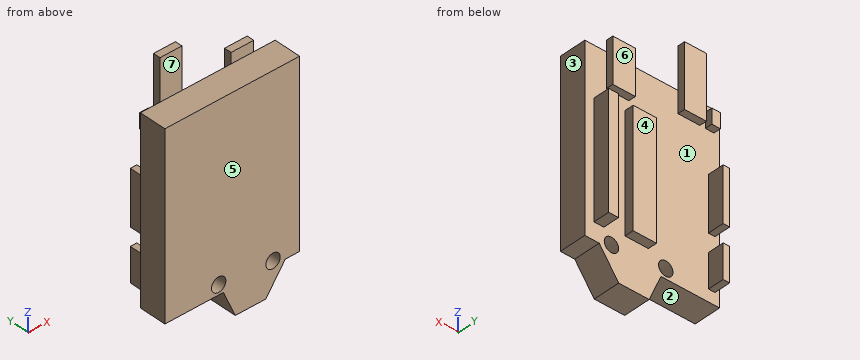
Autodesk Inventor part; units mm, degrees
ref_plane "YZ Plane" through (0, 0, 0) normal (1, 0, 0) x (0, 1, 0)
ref_plane "XZ Plane" through (0, 0, 0) normal (0, 1, 0) x (-1, 0, 0)
ref_plane "XY Plane" through (0, 0, 0) normal (0, 0, 1) x (1, 0, 0)
sketch "Sketch1" plane through (0, 0, 0) normal (0, 1, 0) x (-1, 0, 0)
  line L0 (0, 0) -> (0, -100)
  line L1 (0, 0) -> (75, 0)
  line L2 (75, 0) -> (75, -100)
  line L3 (75, -100) -> (42.4007, -100)
  line L4 (42.4007, -100) -> (35.8215, -115.0757)
  line L5 (35.8215, -115.0757) -> (18.8427, -115.0757)
  line L6 (18.8427, -115.0757) -> (8.0187, -100)
  line L7 (8.0187, -100) -> (0, -100)
  dimension "d0" = 100
  dimension "d1" = 75
extrude "Extrusion1" add sketch "Sketch1" along normal blind 15
sketch "Sketch2" plane through (0, 15, 0) normal (0, 1, 0) x (1, 0, 0)
  line L0 (-72.4361, 34.6384) -> (-68.8116, 34.6384)
  line L1 (-68.8116, 34.6384) -> (-68.8116, 64.722)
  line L2 (-68.8116, 64.722) -> (-72.4361, 64.722)
  line L3 (-72.4361, 64.722) -> (-72.4361, 34.6384)
  line L4 (-72.4361, 74.6291) -> (-68.8116, 74.6291)
  line L5 (-68.8116, 74.6291) -> (-68.8116, 93.3558)
  line L6 (-68.8116, 93.3558) -> (-72.4361, 93.3558)
  line L7 (-72.4361, 93.3558) -> (-72.4361, 74.6291)
  point P0 (0, 0)
extrude "Extrusion2" add sketch "Sketch2" along normal blind 9
sketch "Sketch3" plane through (0, 15, 0) normal (0, 1, 0) x (1, 0, 0)
  line L0 (-10.6109, 27.0955) -> (-5.1141, 27.0955)
  line L1 (-5.1141, 27.0955) -> (-5.1141, 90.5375)
  line L2 (-5.1141, 90.5375) -> (-10.6109, 90.5375)
  line L3 (-10.6109, 90.5375) -> (-10.6109, 27.0955)
  point P0 (0, 0)
extrude "Extrusion3" add sketch "Sketch3" along normal blind 9
sketch "Sketch4" plane through (0, 15, 0) normal (0, 1, 0) x (1, 0, 0)
  line L0 (-24.5308, -5.8613) -> (-11.9398, -5.8613)
  line L1 (-11.9398, -5.8613) -> (-11.9398, 18.8865)
  line L2 (-11.9398, 18.8865) -> (-24.5308, 18.8865)
  line L3 (-24.5308, 18.8865) -> (-24.5308, -5.8613)
  line L4 (-64.0405, -22.7941) -> (-51.8837, -22.7941)
  line L5 (-51.8837, -22.7941) -> (-51.8837, 11.9398)
  line L6 (-51.8837, 11.9398) -> (-64.0405, 11.9398)
  line L7 (-64.0405, 11.9398) -> (-64.0405, -22.7941)
  line L8 (-71.8556, 3.6905) -> (-67.0797, 3.6905)
  line L9 (-67.0797, 3.6905) -> (-67.0797, 11.9398)
  line L10 (-67.0797, 11.9398) -> (-71.8556, 11.9398)
  line L11 (-71.8556, 11.9398) -> (-71.8556, 3.6905)
  point P0 (0, 0)
extrude "Extrusion4" add sketch "Sketch4" along normal blind 4
sketch "Sketch5" plane through (0, 15, 0) normal (0, 1, 0) x (1, 0, 0)
  line L0 (-35.3851, 24.965) -> (-22.3599, 24.965)
  line L1 (-22.3599, 24.965) -> (-22.3599, 89.2226)
  line L2 (-22.3599, 89.2226) -> (-35.3851, 89.2226)
  line L3 (-35.3851, 89.2226) -> (-35.3851, 24.965)
  point P0 (0, 0)
extrude "Extrusion5" add sketch "Sketch5" along normal blind 5
sketch "Sketch6" plane through (0, 15, 0) normal (0, 1, 0) x (1, 0, 0)
  line L0 (-62.9909, 21.9257) -> (-62.9909, 90.0836) construction
  line L1 (-62.9909, 90.0836) -> (-37.1661, 90.0836) construction
  line L2 (-37.1661, 90.0836) -> (-37.1661, 21.9257) construction
  line L3 (-37.1661, 21.9257) -> (-62.9909, 21.9257) construction
  point P0 (0, 0)
sketch "Sketch7" plane through (0, 15, 0) normal (0, 1, 0) x (1, 0, 0)
  point P0 (0, 0)
  point P1 (-14.8096, 97.5183)
  point P2 (-45.0522, 94.6629)
hole "Hole1" at (-14.8096, 15, -97.5183) at (-45.0522, 15, -94.6629) direction (0, -1, 0) diameter 8 end through all
properties part number "arduino now"
Geometry: final body of the model. Coordinates: model frame, mm. Face numbers are marked on the shaded views. A direction names the side the tool comes from. Round coordinates to 2 decimals unless told otherwise and drop trailing zeros. Loops run counter-clockwise (first coordinate to the right, second up) from the corner with the lowest first, then second, coordinate; pieces in that order, holes last. Notation, with made-up numbers: (67.25, -25.5) -> (79.25, -25.5) arc R29 ccw to (79.25, -5.5) -> close; hole circle Ø4 at (-37.75, 72.25). An arc over 180 degrees is marked (long way). One line per question, with ' | ' between items. Start each with the question number.
1. Section A-A on y = 21.75. Output: boundary loops of the cut face in (x, z).
2. Section B-B on x = -28.5. Output: boundary loops of the cut face in (y, z) (3 decimals), and give its area (3 significant figures).
3. Mould query, pull axis X, two halves, no side actions, for the marked faces 1, 2 and 3. Classes: pulls with the +X half, pulls with the -X half, needs draft (parallel to the pull), parting line crosses it, or undercut.
4. Contact query for flat-ended pins moving along their axis: pin 1 (7.5 mm diameter, centred on x = -63, y = 5, fed in from -Z); pin 2 (4.5 mm diameter, centred on y = 17.5, z = -87.5, fed in from -X); pin 3 (1.8 mm diameter, centred on x = -70.5, y = 18, fed in from +Z). Output: stop coordinate, or through.
5. Line query: line 1 along X through (y, z) = (19.75, -60); line 2 along X through (y, z) = (23.25, -37); line 3 along X through (y, z) = (18.5, -2). Output: solid intervals per line, ascending. Write a range as [from, to].
6. Section D-D on z = 14. Output: boundary loops of the cut face in (x, y).
7. Set-up query: the marked faces 4, 5, 6 and 7. Return all of +Z, -Z, +X, -X, +Y, -Y with unobstructed straight access to the full face (end or side cutting, diameter ignored); none if empty.
8. Section C-C on y = 13.5. Output: boundary loops of the cut face in (x, z), and give its area (3 significant figures).
Returned:
1) outline: (-72.44, -93.36) -> (-68.81, -93.36) -> (-68.81, -74.63) -> (-72.44, -74.63) -> close; (-72.44, -64.72) -> (-68.81, -64.72) -> (-68.81, -34.64) -> (-72.44, -34.64) -> close; (-10.61, -90.54) -> (-5.11, -90.54) -> (-5.11, -27.1) -> (-10.61, -27.1) -> close
2) outline: (0, -115.076) -> (15, -115.076) -> (15, -89.223) -> (20, -89.223) -> (20, -24.965) -> (15, -24.965) -> (15, 0) -> (0, 0) -> close | area: 2,050 mm2
3) face 1: undercut | face 2: needs draft | face 3: pulls with the +X half
4) pin 1: stops at z = -100 | pin 2: stops at x = -72.44 | pin 3: stops at z = -3.69
5) line 1: x = [-72.44, -68.81], [-35.39, -22.36], [-10.61, -5.11] | line 2: x = [-72.44, -68.81], [-10.61, -5.11] | line 3: x = [-64.04, -51.88], [-24.53, -11.94]
6) outline: (-64.04, 15) -> (-51.88, 15) -> (-51.88, 19) -> (-64.04, 19) -> close
7) face 4: +Z, -Z, +Y | face 5: +Z, -Z, +X, -X, -Y | face 6: +Z, +X, -X, +Y | face 7: +Z, +X, -X, -Y
8) outline: (-75, -100) -> (-42.4, -100) -> (-35.82, -115.08) -> (-18.84, -115.08) -> (-8.02, -100) -> (0, -100) -> (0, 0) -> (-75, 0) -> close; hole circle Ø8 at (-45.05, -94.66); hole circle Ø8 at (-14.81, -97.52) | area: 7,790 mm2
